Read the model definition and answer for the solid it produces. Units are mm, in the model's axes. Face numbers are marked on the shaded views. A direction names the side the tool comes from. Give positions to 0.01 mm unless a question says otherwise; leave off trailing zeros. Order: outer loops, then holes, each group sorted by start corner. A loop starts at its lowest first (then second) coordinate and runs counter-clockwise, first axis right, second up. Notation, with made-up numbers: (63, 0) - (91, 0) arc R18 ccw to (91, 19) - close; hole circle Ø8 at (40.5, 10). An arc over 180 degrees is marked (long way). Use a Markdown table: item, result. Add a question column.
1. Flat-ended cylindrical pins translate along their axes: P1, Ø1.5, axis at x = -4.5, y = -64.5, coming from the +Z side; P2, Ø12, axis at x = 1, y = -54, coming from the -Z side; P3, Ø4, axis at x = 2.5, z = -3.5, coming from the +Y side. Find the tip coordinate at first contact, or state that the pin passes through.
2. For a pull along Y with two mould halves and no side action, classify the marked faces 1, 2 and 3 as released by +Y, released by -Y, zero draft, split by the parting line, or undercut.
3. Which of the six approach directions +Z, -Z, +X, -X, +Y, -Y give full straight-line access (tool end or side, diameter ignored) to the marked faces 4 and 5?
4. A cutting plane is placed at C-C on y = -56. Determine the outline of the cut face in (x, z), and give its area (3 significant figures).
5. A cutting plane is placed at D-D on x = 2. Determine the outline of the cut face in (y, z).
6. Consider L1, parallel to X at y = -65, z = 6.25; L2, parallel to X at y = -70, z = -4; L3, parallel to X at y = -54.25, z = 9.25. Determine where each line is inside the solid, lowest interval first.
7. A cutting plane is placed at B-B on x = -8.5. Determine the outline of the cut face in (y, z).
8. A cutting plane is placed at A-A on z = -4. Determine the outline of the cut face in (x, y).
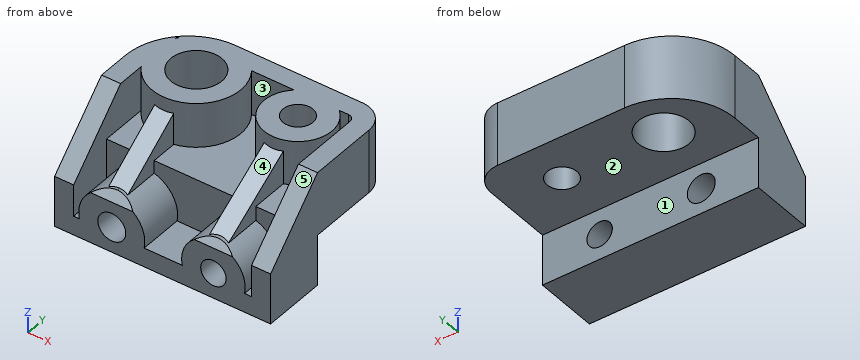
```python
from build123d import *

# Parameters (mm, degrees)
ESQUISSE1_W        = 34
ESQUISSE1_H        = 15
ESQUISSE1_R        = 2.35
ESQUISSE1_R_2      = 4
BOSS_EXTRU_1_DEPTH = 10
ESQUISSE2_W        = 34
ESQUISSE2_H        = 18
ESQUISSE2_R        = 2.2
ESQUISSE2_R_2      = 2
BOSS_EXTRU_2_DEPTH = 10
CHANFREIN2_SIZE    = 10
COQUE1_START       = 3
COQUE1_DEPTH       = 7
COQUE1_START_2     = 1.2
COQUE1_2_OUTLINE_W = 28
COQUE1_2_OUTLINE_H = 7
COQUE1_2_DEPTH     = 1.8
COQUE1_START_3     = -74
COQUE1_3_DEPTH     = 7
CONG_1_R           = 10
CONG_3_R           = 1
CONG_4_R           = 4
NERVURE3_REACH     = 80.746
ESQUISSE4_WALL_W   = 176.697507514
ESQUISSE4_WALL_H   = 3
NERVURE5_REACH     = 80.746
ESQUISSE5_WALL_W   = 178.064946254
ESQUISSE5_WALL_H   = 3


with BuildPart() as part:
    # Esquisse1 → Boss.-Extru.1 (new body)
    with BuildSketch(Plane.XY):
        with Locations((0, -56.5)):
            Rectangle(ESQUISSE1_W, ESQUISSE1_H)
        with Locations((8, -56)):
            Circle(ESQUISSE1_R, mode=Mode.SUBTRACT)
        with Locations((-8, -56)):
            Circle(ESQUISSE1_R_2, mode=Mode.SUBTRACT)
    extrude(amount=BOSS_EXTRU_1_DEPTH)

    # Esquisse2 → Boss.-Extru.2 (add)
    with BuildSketch(Plane.XZ.offset(64)):
        with Locations((0, 1)):
            Rectangle(ESQUISSE2_W, ESQUISSE2_H)
        with Locations(Location((-8, -4, 0), (0, 0, 270))):
            Circle(ESQUISSE2_R, mode=Mode.SUBTRACT)
        with Locations(Location((8, -4, 0), (0, 0, 270))):
            Circle(ESQUISSE2_R_2, mode=Mode.SUBTRACT)
    extrude(amount=BOSS_EXTRU_2_DEPTH)

    # Chanfrein2
    chanfrein2_edges = [part.edges().sort_by_distance(p)[0] for p in [
        (0, -74, 10),
    ]]
    chamfer(chanfrein2_edges, length=CHANFREIN2_SIZE)

    # Coque1: read off the stored shape, not the designer's step
    # Coque1 outline → Coque1 (cut)
    with BuildSketch(Plane.XY.offset(COQUE1_START)):
        with BuildLine():
            Line((14, -74), (14, -52))
            Line((14, -52), (11.552815785, -52))
            ThreePointArc((11.552815785, -52), (8, -61.35), (4.447184215, -52))
            Line((4.447184215, -52), (-2.255437353, -52))
            ThreePointArc((-2.255437353, -52), (-4.19508021, -61.875592344), (-14, -59.605551275))
            Line((-14, -59.605551275), (-14, -74))
            Line((-14, -74), (14, -74))
        make_face()
        with BuildLine():
            ThreePointArc((-14, -52.394448725), (-13.875592344, -52.19508021), (-13.744562647, -52))
            Line((-13.744562647, -52), (-14, -52))
            Line((-14, -52), (-14, -52.394448725))
        make_face()
    extrude(amount=COQUE1_DEPTH, mode=Mode.SUBTRACT)

    # Coque1 2 outline → Coque1 2 (cut)
    with BuildSketch(Plane.XY.offset(COQUE1_START_2)):
        with Locations((0, -70.5)):
            Rectangle(COQUE1_2_OUTLINE_W, COQUE1_2_OUTLINE_H)
    extrude(amount=COQUE1_2_DEPTH, mode=Mode.SUBTRACT)

    # Coque1 3 outline → Coque1 3 (cut)
    with BuildSketch(Plane(origin=(0, 0, 0), x_dir=(1, 0, 0), z_dir=(0, 1, 0)).offset(COQUE1_START_3)):
        with BuildLine():
            ThreePointArc((-2.897059671, 5), (-3.98502802, 0.695457672), (-8, -1.2))
            Line((-8, -1.2), (14, -1.2))
            Line((14, -1.2), (14, 5))
            Line((14, 5), (12.898979486, 5))
            ThreePointArc((12.898979486, 5), (8, -1), (3.101020514, 5))
            Line((3.101020514, 5), (-2.897059671, 5))
        make_face()
        with BuildLine():
            ThreePointArc((-8, -1.2), (-12.01497198, 0.695457672), (-13.102940329, 5))
            Line((-13.102940329, 5), (-14, 5))
            Line((-14, 5), (-14, -1.2))
            Line((-14, -1.2), (-8, -1.2))
        make_face()
    extrude(amount=COQUE1_3_DEPTH, mode=Mode.SUBTRACT)

    # Congé1
    cong_1_edges = [part.edges().sort_by_distance(p)[0] for p in [
        (-17, -49, 5),
    ]]
    fillet(cong_1_edges, radius=CONG_1_R)

    # Congé3
    cong_3_edges = [part.edges().sort_by_distance(p)[0] for p in [
        (14, -52, 6.5),
    ]]
    fillet(cong_3_edges, radius=CONG_3_R)

    # Congé4
    cong_4_edges = [part.edges().sort_by_distance(p)[0] for p in [
        (17, -49, 5),
    ]]
    fillet(cong_4_edges, radius=CONG_4_R)

    # Esquisse4 wall → Nervure3 (add, up to next)
    with BuildSketch(Plane(origin=(-8, -67, 5), x_dir=(0, -0.813733471207, -0.581238193719), z_dir=(0, 0.581238193719, -0.813733471207)), mode=Mode.PRIVATE) as nervure3_sk1:
        Rectangle(ESQUISSE4_WALL_W, ESQUISSE4_WALL_H)
    nervure3_tool1 = extrude(nervure3_sk1.sketch, amount=NERVURE3_REACH, mode=Mode.PRIVATE) - part.part
    add(nervure3_tool1.solids().sort_by_distance((-8, -67, 5))[0])

    # Esquisse5 wall → Nervure5 (add, up to next)
    with BuildSketch(Plane(origin=(8, -66.175, 5), x_dir=(0, -0.842662328893, -0.538442382679), z_dir=(0, 0.538442382679, -0.842662328893)), mode=Mode.PRIVATE) as nervure5_sk1:
        Rectangle(ESQUISSE5_WALL_W, ESQUISSE5_WALL_H)
    nervure5_tool1 = extrude(nervure5_sk1.sketch, amount=NERVURE5_REACH, mode=Mode.PRIVATE) - part.part
    add(nervure5_tool1.solids().sort_by_distance((8, -66.175, 5))[0])


solid = part.part
```
Output values:
| question | item | result |
|---|---|---|
| 1 | P1 | z = 3 |
| 1 | P2 | z = 0 |
| 1 | P3 | y = -64 |
| 2 | face 1 | released by +Y |
| 2 | face 2 | zero draft |
| 2 | face 3 | undercut |
| 3 | face 4 | +Z, -Y |
| 3 | face 5 | +Z, +X, -X, -Y |
| 4 | outline | (-16.54, 0) - (-12, 0) - (-12, 10) - (-16.54, 10) - close; (-4, 0) - (5.65, 0) - (5.65, 10) - (2.65, 10) - (2.65, 3) - (-1, 3) - (-1, 10) - (-4, 10) - close; (10.35, 0) - (17, 0) - (17, 10) - (14, 10) - (14, 3) - (13.35, 3) - (13.35, 10) - (10.35, 10) - close |
| 4 | area | 178 mm² |
| 5 | outline | (-74, -8) - (-64, -8) - (-64, 0) - (-49, 0) - (-49, 10) - (-52, 10) - (-52, 3) - (-67, 3) - (-67, -5) - (-74, -5) - close |
| 6 | L1 | -17 to -14, -9.5 to -6.5, 14 to 17 |
| 6 | L2 | -17 to -14, -13.2 to -10.2, -5.8 to -2.8, 3 to 6, 10 to 13, 14 to 17 |
| 6 | L3 | -15.8 to -11.6, -4.4 to -1.22, 2.94 to 6.43, 9.57 to 13.06, 14 to 17 |
| 7 | outline | (-74, -8) - (-64, -8) - (-64, -6.14) - (-74, -6.14) - close; (-74, -1.86) - (-64, -1.86) - (-64, 0) - (-59.97, 0) - (-59.97, 10) - (-62.98, 10) - (-62.98, 7.87) - (-72.35, 1.18) - (-72.82, 1.18) - (-74, 0) - close; (-52.03, 0) - (-49.11, 0) - (-49.11, 10) - (-52.03, 10) - close |
| 8 | outline | (-17, -74) - (-14, -74) - (-14, -67) - (-13.2, -67) - (-13.2, -74) - (-10.2, -74) - (-10.2, -64) - (-17, -64) - close; (-5.8, -74) - (-2.8, -74) - (-2.8, -67) - (3, -67) - (3, -74) - (6, -74) - (6, -64) - (-5.8, -64) - close; (10, -74) - (13, -74) - (13, -67) - (14, -67) - (14, -74) - (17, -74) - (17, -64) - (10, -64) - close |
